Read the model definition and answer for the solid it produces. Units are mm, in the model's axes. A direction names the side the tool comes from. Coordinates: 2 decimals unless noted, no trailing zeros. Order: outer loops, then holes, each group sorted by start corner. A loop starts at its lowest first (then second) coordinate and runs counter-clockwise, first axis right, second up. Notation, with made-up numbers: (53.5, 39) - (106.5, 39) arc R15 ccw to (106.5, 65) - close; hole circle Ø8 at (64, 11). An arc over 180 degrees is marked (long way). Answer as a JSON object with one key per item and string values. Group by question number.
from build123d import *

# Parameters (mm, degrees)
SKETCH2_R          = 50
CUT_EXTRUDE1_DEPTH = 436.889894354


with BuildPart() as part:
    # Sketch1 → Revolve1 (revolve)
    with BuildSketch(Plane.XY, mode=Mode.PRIVATE) as revolve1_sk:
        Polygon((0, 0), (0, 300), (25, 300), (25, 290), (75, 290), (75, 300), (100, 300), (100, 0), align=None)
    revolve(revolve1_sk.sketch.rotate(Axis((0, 0, 0), (1, 0, 0)), 90), axis=Axis((0, 0, 0), (1, 0, 0)))

    # Sketch2 → Cut-Extrude1 (cut, through all)
    with BuildSketch(Plane.ZY):
        Circle(SKETCH2_R)
    extrude(amount=-CUT_EXTRUDE1_DEPTH, mode=Mode.SUBTRACT)


solid = part.part
1. A cutting plane is placed at D-D on y = 141.5. Write down the section's boundary in (x, z).
2. For a pull along X with two mould halves and no side action, classify faces 1 (the flat face through (0, 62, 4)), 2 (the flat face through (75, -246, 157)), 3 (the cylindrical face through (12.675, 266.152, 138.432)) as pulls with the +X half, pulls with the -X half, needs draft (parallel to the pull), parting line crosses it, or undercut.
3. Straight lines are drawn through the part: L1, parallel to Y at x = 79, z = 0; L2, parallel to Y at x = 37.5, z = 0; L3, parallel to X at y = -125.5, z = 262. For each, find the intervals that lie inside material, in ascending order.
4. Given pin 1 (5 mm diameter, centred on x = 32, z = 38, fed in from -Y); pin 2 (2 mm diameter, centred on x = 36.5, y = 8.5, fed in from -Z); pin 3 (5 mm diameter, centred on y = -46, z = 222.5, fed in from -X); pin 4 (8 mm diameter, centred on x = 10.5, z = 118, fed in from -Y), each flat-ended and moving along its own axis, determine where each tip first touches the part or whether it passes through.
5. For faces 4 (the cylindrical face through (50.35, 257.28, 133.82)), 5 (the cylindrical face through (87.675, 266.152, 138.432)), determine the directions among +Z, -Z, +X, -X, +Y, -Y from which every point of the face is accessible in a straight line to the end or side of a thin tool.
6. A cutting plane is placed at C-C on x = 85. Write down the section's boundary in (y, z), and give its area (3 significant figures).
7. A cutting plane is placed at A-A on y = 0. Write down the section's boundary in (x, z), and give its area (3 significant figures).
Derived:
{
 "1": {"outline": "(0, -264.53) - (25, -264.53) - (25, -253.14) - (75, -253.14) - (75, -264.53) - (100, -264.53) - (100, 264.53) - (75, 264.53) - (75, 253.14) - (25, 253.14) - (25, 264.53) - (0, 264.53) - close"},
 "2": {"face 1": "pulls with the -X half", "face 2": "undercut", "face 3": "needs draft"},
 "3": {"L1": "y = -300 to -50, 50 to 300", "L2": "y = -290 to -50, 50 to 290", "L3": "x = 0 to 25, 75 to 100"},
 "4": {"pin 1": "stops at y = -287.82", "pin 2": "stops at z = -289.9", "pin 3": "stops at x = 0", "pin 4": "stops at y = -277.5"},
 "5": {"face 4": "none", "face 5": "+X, -X"},
 "6": {"outline": "circle Ø600 at (0, 0); hole circle Ø100 at (0, 0)", "area": "275,000 mm2"},
 "7": {"outline": "(0, -300) - (25, -300) - (25, -290) - (75, -290) - (75, -300) - (100, -300) - (100, -50) - (0, -50) - close; (0, 50) - (100, 50) - (100, 300) - (75, 300) - (75, 290) - (25, 290) - (25, 300) - (0, 300) - close", "area": "49,000 mm2"}
}
